Geometry: final body of the model. Coordinates: model frame, mm. Face numbers are marked on the shaded views. Give positions to 0.01 mm unless a question says otherwise; leave off trailing zeros. Write each loop counter-clockwise with the first axis right and the second up, starting at its lowest first coordinate (ties: lowest second). Pieces come first, ordered by that corner, then holes. Notation, with made-up numbers: M 44.5,3.25 L 85.5,3.25 A18 cw 85.5,15.25 Z; hole C 48.25,30.25 d1. An arc over 180 degrees is marked long. One line per question, with ' | ' between items.
Autodesk Inventor part; units mm, degrees
ref_plane "Arbeitsebene1" through (-25, 0, 65) normal (0, 0, 1) x (1, 0, 0)
ref_plane "YZ Plane" through (0, 0, 0) normal (1, 0, 0) x (0, 1, 0)
ref_plane "XZ Plane" through (0, 0, 0) normal (0, 1, 0) x (-1, 0, 0)
sketch "Skizze1" plane through (0, 0, 0) normal (0, 1, 0) x (-1, 0, 0)
  line L0 (25, -15) -> (-25, -15)
  line L1 (-25, -15) -> (-25, 15)
  line L2 (-25, 15) -> (25, 15)
  line L3 (25, 15) -> (25, -15)
  line L4 (35, 0) -> (-35, 0)
  line L5 (0, -38.6491) -> (0, 126.8947)
  point P0 (0, 0)
  dimension "d0" = 50
  dimension "d1" = 30
extrude "Extrusion1" add sketch "Skizze1" along normal blind 20
ref_plane "Arbeitsebene1" through (-25, 0, 65) normal (0, 0, 1) x (1, 0, 0)
sketch "Skizze8" plane through (-25, 0, 15) normal (0, 0, 1) x (1, 0, 0)
  ellipse E0 centre (25, 10) end of major axis (45, 10) minor radius 7
  line L0 (50, 0) -> (50, 20)
  line L1 (50, 10) -> (0, 10)
  line L2 (0, 0) -> (0, 20)
  line L3 (50, 0) -> (0, 0)
  line L4 (0, 10) -> (50, 10)
  point P0 (25, 0)
  dimension "d25" = 20
  dimension "d26" = 7
  dimension "d38" = 10
sketch "Skizze9" plane through (0, 0, 0) normal (1, 0, 0) x (0, 1, 0)
  line L0 (0, 15) -> (20, 15)
  line L1 (-90, 68) -> (-60, 68)
  line L2 (-60, 68) -> (-90, 68)
  spline S0 degree 4 poles (10, 15) (9.5803, 71.5574) (15.9295, 84.5237) (-76.3854, 91.7546) (-75, 68) knots 0 0 0 0 0 1 1 1 1 1
  line L3 (10.1796, -9.2022) -> (9.8204, 39.2022) construction
  arc A0 (10.5195, 34.3212) -> (10.8062, -4.3113) centre (291.7825, 17.0911) ccw construction
  point P0 (0, 0)
  point P1 (-1.3064, 69.8283)
  point P2 (-48.271, 81.8124)
sweep "Sweeping5" add profiles "Skizze8" path "Skizze9" path curves S0 contours L1 E0 | E0 L1
properties part number "_3D-Druck"
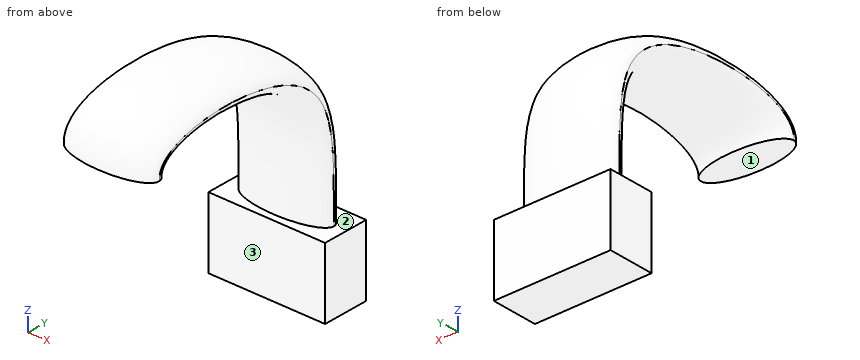
(1) First-contact query: P1, Ø12, axis at x = -6, z = 77, coming from the +Y side; P2, Ø10, axis at x = 0.5, y = 8, coming from the +Z side; P3, Ø4, axis at x = 17, y = -28.5, coming from the -Z side. Flat tips, straight axial feed; report the tip coordinate or a pass-through.
Working result:
P1: stops at y = 6.77 | P2: stops at z = 75.37 | P3: stops at z = 76.31
(2) Cut plane A-A, the plane z = 7. Return loops of the section in (x, y), then the cut area to 3 significant figures.
Working result:
outline: M -25,0 L 25,0 L 25,20 L -25,20 Z | area: 1,000 mm^2
(3) Material intervals for L1, parallel to Y at x = 16.5, z = 6.5; L2, parallel to Z at x = -7, y = -29.5; L3, parallel to Z at x = 17, y = -61, sorted ascending. Write a range as [from, to].
Working result:
L1: y = [0, 20] | L2: z = [74.57, 87.81] | L3: z = [76.04, 83.66]
(4) Draft query along Y for the marked faces 1, 2 and 3. Return one class per face: released by +Y, released by -Y, zero draft, split by the parting line, or undercut.
Working result:
face 1: undercut | face 2: zero draft | face 3: released by -Y
